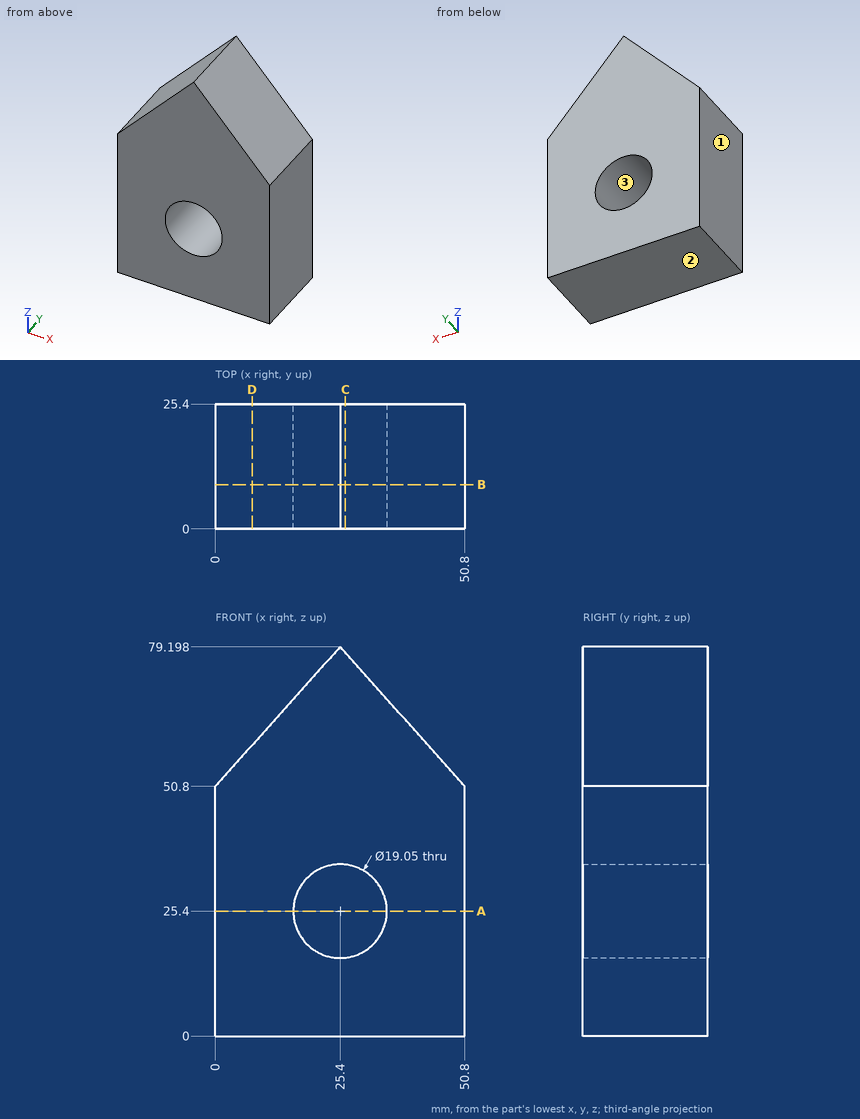
Geometry: see drawing. Coordinates: mm, zero at the bounding-box minimum. Give positions to 0.01 mm unless a question says otherwise; leave off trailing zeros. Order: outer loops, then holes, each group sorted by start corner. A loop starts at its lowest first (then second) coordinate and runs counter-clockwise, first axis right, second up. Notation, with made-up numbers: (-12, 46.25) -> (13, 46.25) arc R22 cw to (13, 70.25) -> close; hole circle Ø6 at (46, 68). An arc over 180 degrees is marked (long way). Write each question's results on one line, items separated by ' | '.
1) First-contact query: pin 1 Ø1 at (y, z) = (15, 71) entering from -X. Flat tip, straight axial feed; report the tip coordinate or a pass-through.
Geometry says:
pin 1: stops at x = 17.62
2) Cut plane B-B (y = 9). Output: boundary loops of the cut face in (x, z) (3 decimals), and give its area (3 significant figures).
Geometry says:
outline: (0, 0) -> (50.8, 0) -> (50.8, 50.8) -> (25.4, 79.198) -> (0, 50.8) -> close; hole circle Ø19.05 at (25.4, 25.4) | area: 3,020 mm²
3) Draft query along Z for the marked faces 1, 2 and 3. Return one class per face: released by +Z, released by -Z, zero draft, split by the parting line, or undercut.
Geometry says:
face 1: zero draft | face 2: released by -Z | face 3: undercut
4) Line query: line 1 along X through (y, z) = (18.75, 25); line 2 along Z through (x, y) = (3.5, 9.5); line 3 along Z through (x, y) = (20.5, 23.75). Output: solid intervals per line, ascending.
Geometry says:
line 1: x = 0 to 15.88, 34.92 to 50.8 | line 2: z = 0 to 54.71 | line 3: z = 0 to 17.23, 33.57 to 73.72
5) Cut plane C-C (x = 26.5). Output: boundary loops of the cut face in (y, z), and give its area (3 significant figures).
Geometry says:
outline: (0, 0) -> (25.4, 0) -> (25.4, 15.94) -> (0, 15.94) -> close; (0, 34.86) -> (25.4, 34.86) -> (25.4, 77.97) -> (0, 77.97) -> close | area: 1,500 mm²
6) Cut plane D-D (x = 7.5). Output: boundary loops of the cut face in (y, z).
Geometry says:
outline: (0, 0) -> (25.4, 0) -> (25.4, 59.19) -> (0, 59.19) -> close
7) Cut plane A-A (z = 25.4). Output: boundary loops of the cut face in (x, y) (3 decimals), and give its area (3 significant figures).
Geometry says:
outline: (0, 0) -> (15.875, 0) -> (15.875, 25.4) -> (0, 25.4) -> close; (34.925, 0) -> (50.8, 0) -> (50.8, 25.4) -> (34.925, 25.4) -> close | area: 806 mm²
